```python
from build123d import *

# Parameters (mm, degrees)
BOSS_EXTRUDE1_DEPTH                                 = 3
BOSS_EXTRUDE2_DEPTH                                 = 4
SKETCH3_W                                           = 6
SKETCH3_H                                           = 5
BOSS_EXTRUDE3_DEPTH                                 = 3.5
FILLET1_R                                           = 3
FILLET3_R                                           = 10
CSK_FOR_M3_COUNTERSUNK_FLAT_HEAD_SCREW1_D           = 3.4
CSK_FOR_M3_COUNTERSUNK_FLAT_HEAD_SCREW1_DEPTH       = 20
CSK_FOR_M3_COUNTERSUNK_FLAT_HEAD_SCREW1_CSINK_D     = 6.7
CSK_FOR_M3_COUNTERSUNK_FLAT_HEAD_SCREW1_CSINK_ANGLE = 90
CSK_FOR_M3_COUNTERSUNK_FLAT_HEAD_SCREW1_TIP         = 1.021463052
CUT_EXTRUDE1_DEPTH                                  = 10
FILLET4_R                                           = 1


with BuildPart() as part:
    # Sketch1 → Boss-Extrude1 (new body)
    with BuildSketch(Plane.XY):
        with BuildLine():
            Line((-10, -10), (10, -10))
            ThreePointArc((10, -10), (13.535533906, -8.535533906), (15, -5))
            Line((15, -5), (15, 5))
            ThreePointArc((15, 5), (13.535533906, 8.535533906), (10, 10))
            Line((10, 10), (-10, 10))
            ThreePointArc((-10, 10), (-13.535533906, 8.535533906), (-15, 5))
            Line((-15, 5), (-15, -5))
            ThreePointArc((-15, -5), (-13.535533906, -8.535533906), (-10, -10))
        make_face()
    extrude(amount=BOSS_EXTRUDE1_DEPTH)

    # Sketch2 → Boss-Extrude2 (add, symmetric)
    with BuildSketch(Plane(origin=(0, 0, 0), x_dir=(1, 0, 0), z_dir=(0, 1, 0))):
        Polygon((15, 0), (15, -14.95), (34, -14.95), (34, -18.45), (9, -18.45), (9, 0), align=None)
    extrude(amount=BOSS_EXTRUDE2_DEPTH, both=True)

    # Sketch3 → Boss-Extrude3 (add)
    with BuildSketch(Plane.XY.offset(18.45)):
        with Locations((31, 6.5)):
            Rectangle(SKETCH3_W, SKETCH3_H)
        with Locations((31, -6.5)):
            Rectangle(SKETCH3_W, SKETCH3_H)
    extrude(amount=-BOSS_EXTRUDE3_DEPTH)

    # Fillet1
    fillet1_edges = [part.edges().sort_by_distance(p)[0] for p in [
        (12, 4, 3),
        (9, 0, 3),
        (12, -4, 3),
        (9, 0, 18.45),
    ]]
    fillet(fillet1_edges, radius=FILLET1_R)

    # Fillet3
    fillet3_edges = [part.edges().sort_by_distance(p)[0] for p in [
        (15, 0, 14.95),
    ]]
    fillet(fillet3_edges, radius=FILLET3_R)

    # CSK for M3 Countersunk Flat Head Screw1
    with Locations(Plane(origin=(0, 5, 3), x_dir=(1, 0, 0), z_dir=(0, 0, 1))):
        with Locations((0, 0), (0, -10)):
            CounterSinkHole(CSK_FOR_M3_COUNTERSUNK_FLAT_HEAD_SCREW1_D / 2, CSK_FOR_M3_COUNTERSUNK_FLAT_HEAD_SCREW1_CSINK_D / 2, depth=CSK_FOR_M3_COUNTERSUNK_FLAT_HEAD_SCREW1_DEPTH, counter_sink_angle=CSK_FOR_M3_COUNTERSUNK_FLAT_HEAD_SCREW1_CSINK_ANGLE)
            with Locations((0, 0, -(CSK_FOR_M3_COUNTERSUNK_FLAT_HEAD_SCREW1_DEPTH + CSK_FOR_M3_COUNTERSUNK_FLAT_HEAD_SCREW1_TIP / 2))):  # 118° drill point
                Cone(0, CSK_FOR_M3_COUNTERSUNK_FLAT_HEAD_SCREW1_D / 2, CSK_FOR_M3_COUNTERSUNK_FLAT_HEAD_SCREW1_TIP, mode=Mode.SUBTRACT)

    # Sketch6 → Cut-Extrude1 (cut)
    with BuildSketch(Plane.XY.offset(3)):
        Polygon((-3.179643035, 2.933019371), (-4.626512789, 2.933019371), (-4.626512789, -0.799365029), (-4.67476253, -0.799365029), (-11.458554614, 3.29759659), (-12.490123019, 3.29759659), (-12.490123019, -3.072836961), (-10.93658358, -3.072836961), (-10.93658358, 0.975645142), (-10.888042331, 0.975645142), (-4.253108018, -3.036364149), (-3.179643035, -3.036364149), align=None)
    extrude(amount=-CUT_EXTRUDE1_DEPTH, mode=Mode.SUBTRACT)

    # Fillet4
    fillet4_edges = [part.edges().sort_by_distance(p)[0] for p in [
        (34, 9, 16.7),
        (28, 9, 16.7),
        (34, -9, 16.7),
        (28, -9, 16.7),
    ]]
    fillet(fillet4_edges, radius=FILLET4_R)


solid = part.part
```
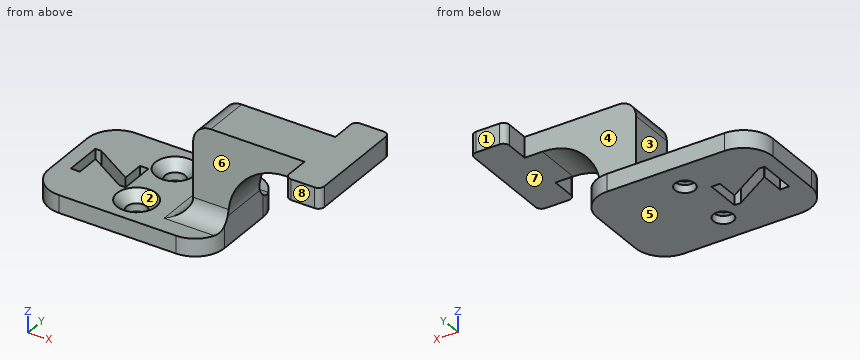
Work out the finished part from the listing and answer in its coordinate system (mm). Face numbers are marked on the shaded views. A direction names the side the tool comes from. Give positions to 0.01 mm unless a question says otherwise; leave off trailing zeros. Write each loop counter-clockwise with the first axis right and the second up, starting at its lowest first coordinate (ties: lowest second). Pieces come first, ordered by that corner, then holes.
(1) The part is cut by section C-C on z = 16. Write down the section's boundary in (x, y), plus the area to 3 significant figures.
Final values:
outline: (9.05, -4) - (28, -4) - (28, -8) arc R1 ccw to (29, -9) - (33, -9) arc R1 ccw to (34, -8) - (34, 8) arc R1 ccw to (33, 9) - (29, 9) arc R1 ccw to (28, 8) - (28, 4) - (9.05, 4) - close
area: 259 mm2
(2) The part is cut by section B-B on x = -7. Write down the section's boundary in (y, z), plus the area to 3 significant figures.
Final values:
outline: (-10, 0) - (-1.38, 0) - (-1.38, 3) - (-10, 3) - close; (0.6, 0) - (10, 0) - (10, 3) - (0.6, 3) - close
area: 54.1 mm2
(3) The part is cut by section A-A on x = 0. Write down the section's boundary in (y, z).
Final values:
outline: (-10, 0) - (-6.7, 0) - (-6.7, 1.35) - (-8.35, 3) - (-10, 3) - close; (-3.3, 0) - (3.3, 0) - (3.3, 1.35) - (1.65, 3) - (-1.65, 3) - (-3.3, 1.35) - close; (6.7, 0) - (10, 0) - (10, 3) - (8.35, 3) - (6.7, 1.35) - close
(4) The mould has two halves that part along Y. Classify the marked faces 1, 2 and 3: pulls with the +Y half, pulls with the -Y half, needs draft (parallel to the pull), parting line crosses it, or undercut.
Final values:
face 1: pulls with the +Y half
face 2: undercut
face 3: needs draft
(5) Which of the six approach directions +Z, -Z, +X, -X, +Y, -Y give full straight-line access (tool end or side, diameter ignored) to the marked faces 4, 5, 6, 7 and 8?
Final values:
face 4: +Z, -X, +Y
face 5: -Z, +X, -X, +Y, -Y
face 6: +Z, -X, -Y
face 7: -Z, +X, +Y, -Y
face 8: +Z, -Z, +X, -X, -Y
(6) Straight lines are drawn through the part: line 1 (Y direction, x = 0, z = 0.35); line 2 (X direction, y = -5, z = 0.45); line 3 (X direction, y = -4.75, z = 17.25). For each, find the intervals that lie inside material, in ascending order.
Final values:
line 1: y = -10 to -6.7, -3.3 to 3.3, 6.7 to 10
line 2: x = -15 to -1.7, 1.7 to 15
line 3: x = 28 to 34
(7) Flat-ended cylindrical pins translate along their axes: pin 1 Ø6 at (x, y) = (-7, 0) entering from +Z; pin 2 Ø4 at (y, z) = (1.5, 2) entering from +X; pin 3 Ø4 at (y, z) = (-4, 12) entering from +X; pin 4 Ø1.5 at (y, z) = (-5.5, 12) entering from -X. Find the tip coordinate at first contact, or state that the pin passes through.
Final values:
pin 1: stops at z = 3
pin 2: stops at x = 15
pin 3: stops at x = 20.75
pin 4: passes through
